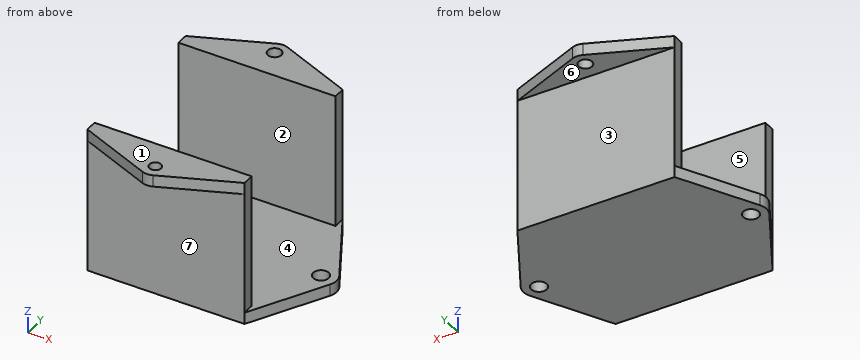
Autodesk Inventor part; units mm, degrees
ref_plane "YZ Plane" through (0, 0, 0) normal (1, 0, 0) x (0, 1, 0)
ref_plane "XZ Plane" through (0, 0, 0) normal (0, 1, 0) x (-1, 0, 0)
ref_plane "XY Plane" through (0, 0, 0) normal (0, 0, 1) x (1, 0, 0)
sketch "Sketch1" plane through (0, 0, 0) normal (0, 0, 1) x (1, 0, 0)
  circle A0 centre (0, 0) radius 1.75
  line L0 (0, 0) -> (0, -50.75)
  circle A1 centre (0, -50.75) radius 1.5
  line L1 (0, 0) -> (0, -7.5)
  line L2 (0, -7.5) -> (0, -4.5)
  line L3 (-20, -7.5) -> (20, -7.5)
  line L4 (-20, -4.5) -> (20, -4.5)
  circle A2 centre (0, 0) radius 3.5
  line L5 (-20, -4.5) -> (-1.34, 3.2333)
  line L6 (20, -4.5) -> (1.34, 3.2333)
  line L7 (-20, -4.5) -> (-20, -7.5)
  line L8 (20, -4.5) -> (20, -7.5)
  line L9 (0, -50.75) -> (0, -43.25)
  line L10 (0, -43.25) -> (0, -46.25)
  line L11 (-20, -43.25) -> (20, -43.25)
  line L12 (-20, -46.25) -> (20, -46.25)
  circle A3 centre (0, -50.75) radius 3.5
  line L13 (-20, -43.25) -> (-20, -46.25)
  line L14 (-20, -46.25) -> (-1.34, -53.9833)
  line L15 (20, -43.25) -> (20, -46.25)
  line L16 (20, -46.25) -> (1.34, -53.9833)
  dimension "d0" = 3.5
  dimension "d1" = 50.75
  dimension "d2" = 3
  dimension "d3" = 7.5
  dimension "d4" = 3
  dimension "d5" = 40
  dimension "d6" = 40
  dimension "d7" = 7
  dimension "d8" = 7.5
  dimension "d9" = 3
  dimension "d10" = 40
  dimension "d11" = 40
  dimension "d12" = 7
extrude "Extrusion1" add sketch "Sketch1" along normal blind 3
extrude "Extrusion2" add sketch "Sketch1" against normal blind 31.5 contours L4 L8 L3 L0 | L0 L3 L7 L4 | L11 L15 L12 L0 | L0 L12 L13 L11
sketch "Sketch2" plane through (0, 0, -31.5) normal (0, 0, -1) x (-1, 0, 0)
  line L0 (-20, -7.5) -> (-20, -4.5)
  line L1 (-20, -4.5) -> (20, -4.5)
  line L2 (20, -4.5) -> (20, -46.25)
  line L3 (20, -46.25) -> (-20, -46.25)
  line L4 (-20, -46.25) -> (-20, -4.5)
  line L5 (20, -7.5) -> (-20, -7.5)
  line L6 (0, -7.5) -> (0, -25.375)
  line L7 (-20, -43.25) -> (20, -43.25)
  line L8 (-27, -25.375) -> (27, -25.375)
  circle A0 centre (-27, -25.375) radius 4
  circle A1 centre (-27, -25.375) radius 2
  circle A2 centre (27, -25.375) radius 4
  circle A3 centre (27, -25.375) radius 2
  line L9 (-20, -4.5) -> (-30.4983, -23.4354)
  line L10 (-1.34, -53.9833) -> (-20, -46.25)
  line L11 (-20, -46.25) -> (-30.4983, -27.3146)
  line L12 (20, -46.25) -> (30.4983, -27.3146)
  line L13 (20, -4.5) -> (30.4983, -23.4354)
  point P0 (0, 0)
  dimension "d17" = 17.875
  dimension "d18" = 54
  dimension "d19" = 8
  dimension "d20" = 4
  dimension "d21" = 8
  dimension "d22" = 4
extrude "Extrusion3" add sketch "Sketch2" along normal blind 3
properties part number "Mount"
The listing builds one solid part. Answer for the finished solid, in the listing's coordinates (mm). Face numbers are marked on the shaded views. A direction names the side the tool comes from. Give positions to 0.01 mm unless a question says otherwise; leave off trailing zeros. Order: outer loops, then holes, each group sorted by start corner. A loop starts at its lowest first (then second) coordinate and runs counter-clockwise, first axis right, second up. Notation, with made-up numbers: (61.5, 68) -> (73.5, 68) arc R20 ccw to (73.5, 100) -> close; hole circle Ø6 at (73, 19.25). An arc over 180 degrees is marked (long way). Put each result on its own line as item: value.
Item 1: For a pull along Y with two mould halves and no side action, classify the marked faces 4, 5, 6 and 7 as released by +Y, released by -Y, zero draft, split by the parting line, or undercut.
Established:
face 4: undercut
face 5: undercut
face 6: zero draft
face 7: released by -Y
Item 2: Straight lines are drawn through the part: line 1 (Y direction, x = 0, z = 0.9); line 2 (Y direction, x = 15, z = -14); line 3 (Z direction, x = -5, y = -47). For each, find the intervals that lie inside material, in ascending order.
Established:
line 1: y = -54.25 to -52.25, -49.25 to -43.25, -7.5 to -1.75, 1.75 to 3.5
line 2: y = -46.25 to -43.25, -7.5 to -4.5
line 3: z = 0 to 3
Item 3: Given P1, Ø10, axis at x = 13, z = -28.5, coming from the +Y side; P2, Ø6.5, axis at x = -3, y = -52, coming from the -Z side; P3, Ø8, axis at x = -5.5, y = -32.5, coming from the +Z side, each flat-ended and moving along its own axis, determine where each tip first touches the part or whether it passes through.
Established:
P1: stops at y = -4.5
P2: stops at z = 0
P3: stops at z = -31.5
Item 4: A cutting plane is placed at D-D on x = -10. Give the vertices of the cut face in (y, z).
Established:
outline: (-50.39, 0) -> (-46.25, 0) -> (-46.25, -34.5) -> (-4.5, -34.5) -> (-4.5, 0) -> (-0.36, 0) -> (-0.36, 3) -> (-7.5, 3) -> (-7.5, -31.5) -> (-43.25, -31.5) -> (-43.25, 3) -> (-50.39, 3) -> close
Item 5: For the marked faces 1, 2 and 3, determine the directions among +Z, -Z, +X, -X, +Y, -Y from which every point of the face is accessible in a straight line to the end or side of a thin tool.
Established:
face 1: +Z, +X, -X, +Y, -Y
face 2: +Z, +X, -X
face 3: -Z, +X, -X, +Y
Item 6: A cutting plane is placed at A-A on x = 0. Give the vertices of the cut face in (y, z).
Established:
outline: (-54.25, 0) -> (-52.25, 0) -> (-52.25, 3) -> (-54.25, 3) -> close; (-49.25, 0) -> (-46.25, 0) -> (-46.25, -34.5) -> (-4.5, -34.5) -> (-4.5, 0) -> (-1.75, 0) -> (-1.75, 3) -> (-7.5, 3) -> (-7.5, -31.5) -> (-43.25, -31.5) -> (-43.25, 3) -> (-49.25, 3) -> close; (1.75, 0) -> (3.5, 0) -> (3.5, 3) -> (1.75, 3) -> close
Item 7: A cutting plane is placed at B-B on z = -23. Give the vertices of the cut face in (x, y).
Established:
outline: (-20, -46.25) -> (20, -46.25) -> (20, -43.25) -> (-20, -43.25) -> close; (-20, -7.5) -> (20, -7.5) -> (20, -4.5) -> (-20, -4.5) -> close
Item 8: A cutting plane is placed at C-C on x = 26. Give the vertices of the cut face in (y, z), plus the area to 3 significant figures.
Established:
outline: (-35.43, -34.5) -> (-27.11, -34.5) -> (-27.11, -31.5) -> (-35.43, -31.5) -> close; (-23.64, -34.5) -> (-15.32, -34.5) -> (-15.32, -31.5) -> (-23.64, -31.5) -> close
area: 49.9 mm^2
